For this review, take the finished solid that the model builds, in its own axes (mm). Round coordinates to 2 decimals unless told otherwise and drop trailing zeros. Write each loop counter-clockwise with the first axis right and the second up, starting at its lowest first coordinate (ties: lowest second). Pieces come first, ordered by that corner, then holes. Notation, with made-up numbers: (50.5, 52.25) -> (81.5, 52.25) arc R8 cw to (81.5, 64.25) -> close; hole circle Ø10 at (-8.75, 85.25). An arc over 180 degrees is marked (long way). Write each question's results on one line, items separated by ' | '. Start each with the question number.
Item 1: Add section C-C (x = 88). State the section outline as (y, z) points, plus the area to 3 significant figures.
Item 2: Add section A-A (z = 3.4). State the section outline as (x, y) points, plus the area to 3 significant figures.
Item 3: To check wall thickness, follow line 1 along Y through (x, z) = (5.5, 2.9); line 2 along X through (y, z) = (5.25, 1.7); line 3 along Y through (x, z) = (96, 2.95). State the ranges of each line that lie inside material, in increasing order.
Item 4: Add section B-B (y = 7). State the section outline as (x, z) points, plus the area to 3 significant figures.
Item 5: Clearance check with flat-ended pins moving along their axes: pin 1 (2 mm diameter, centred on x = 29, z = 1.5, fed in from -Y); pin 2 (3 mm diameter, centred on x = 65, z = 3.5, fed in from +Y); pin 3 (2 mm diameter, centred on x = 13.5, z = 0.5, fed in from -Y). State where each tip first meets the part, or that it passes through.
Autodesk Inventor part; units mm, degrees
ref_plane "YZ Plane" through (0, 0, 0) normal (1, 0, 0) x (0, 1, 0)
ref_plane "XZ Plane" through (0, 0, 0) normal (0, 1, 0) x (-1, 0, 0)
ref_plane "XY Plane" through (0, 0, 0) normal (0, 0, 1) x (1, 0, 0)
sketch "スケッチ1" plane through (0, 0, 0) normal (0, 0, 1) x (1, 0, 0)
  circle A0 centre (0, 5) radius 1.55
  circle A1 centre (0, -5) radius 1.55
  line L0 (0, 5) -> (0, -5) construction
  line L1 (0, 0) -> (100, 0) construction
  circle A2 centre (100, 0) radius 1.55
  line L2 (-5, 10) -> (-5, -10)
  line L3 (-5, -10) -> (5, -10)
  line L4 (5, -10) -> (100.2521, -5.9947)
  line L5 (-5, 10) -> (5, 10)
  line L6 (5, 10) -> (100.2521, 5.9947)
  arc A3 (100.2521, -5.9947) -> (100.2521, 5.9947) centre (100, 0) ccw
  circle A4 centre (0, 5) radius 3 construction
  circle A5 centre (0, 5) radius 5 construction
  line L7 (5, 10) -> (5, -10) construction
  point P0 (-5, 0)
  dimension "d0" = 10
  dimension "d1" = 3.1
  dimension "d2" = 3.1
  dimension "d3" = 100
  dimension "d4" = 6
  dimension "d5" = 6
  dimension "d6" = 2
extrude "押し出し1" add sketch "スケッチ1" along normal blind 5
sketch "スケッチ5" plane through (0, 0, 5) normal (0, 0, 1) x (1, 0, 0)
  circle A0 centre (100, 0) radius 1.55
  circle A1 centre (100, 0) radius 1.55
  circle A2 centre (0, -5) radius 1.55
  circle A3 centre (0, -5) radius 1.55
  circle A4 centre (0, 5) radius 1.55
  circle A5 centre (0, 5) radius 1.55
  point P0 (0, 0)
extrude "押し出し5" add sketch "スケッチ5" against normal up to surface (5 mm away)
properties part number "胴体_サブフレーム_1_12" material "アセタール樹脂、黒"
Responses:
1) outline: (-6.51, 0) -> (6.51, 0) -> (6.51, 5) -> (-6.51, 5) -> close | area: 65.1 mm^2
2) outline: (-5, -10) -> (5, -10) -> (100.25, -5.99) arc R6 ccw to (100.25, 5.99) -> (5, 10) -> (-5, 10) -> close | area: 1,780 mm^2
3) line 1: y = -9.98 to 9.98 | line 2: x = -5 to 102.9 | line 3: y = -6.17 to 6.17
4) outline: (-5, 0) -> (76.34, 0) -> (76.34, 5) -> (-5, 5) -> close | area: 407 mm^2
5) pin 1: stops at y = -9.03 | pin 2: stops at y = 7.54 | pin 3: stops at y = -9.68
